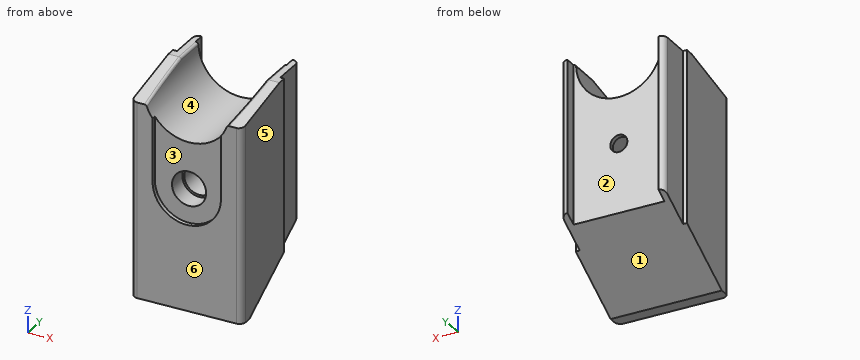
from build123d import *

# Parameters (mm, degrees)
F1_DEPTH  = 26
F2_R      = 10
F2_R_2    = 2
F3_DEPTH  = 26
F4_R      = 3.5
F4_R_2    = 2
F5_DEPTH  = 22.3
F6_R      = 4
F6_R_2    = 3.5
F7_DEPTH  = 5.4
F8_R      = 0.6
F9_W      = 0.9285709113
F9_H      = 8
F10_DEPTH = 61.5
F11_R     = 1.4
F12_W     = 21.2637362675
F12_H     = 42.3296708614
F13_DEPTH = 2.6
F15_DEPTH = 1


with BuildPart() as f1:
    # F0 (on Right) → F1 (new body)
    with BuildSketch(Plane.YZ):
        Polygon((-10, 28.8693108244), (-26, 25.475452911), (-26, -20.1306891756), (-23, -20.1306891756), (0, -6.8516329843), (0, 28.8693108244), align=None)
    extrude(amount=F1_DEPTH)

    # F2 (on face) → F3 (cut)
    with BuildSketch(Plane.XZ.offset(26)):
        with Locations((13, 28.6730788648)):
            Circle(F2_R)
        with Locations((13, 7.8693108244)):
            Circle(F2_R_2)
    extrude(amount=-F3_DEPTH, mode=Mode.SUBTRACT)

    # F4 (on face) → F5 (cut)
    with BuildSketch(Plane.XZ.offset(26)):
        with Locations((13, 7.8693108244)):
            Circle(F4_R)
        with Locations((13, 7.8693108244)):
            Circle(F4_R_2, mode=Mode.SUBTRACT)
    extrude(amount=-F5_DEPTH, mode=Mode.SUBTRACT)

    # F6 (on face) → F7 (cut)
    with BuildSketch(Plane.XZ.offset(26)):
        with Locations((13, 7.8693108244)):
            Circle(F6_R)
        with Locations((13, 7.8693108244)):
            Circle(F6_R_2, mode=Mode.SUBTRACT)
    extrude(amount=-F7_DEPTH, mode=Mode.SUBTRACT)

    # F8
    f8_edges = [f1.edges().sort_by_distance(p)[0] for p in [
        (3.113398, -18.00473, 27.171379),
        (22.999519, -10.462557, 28.771195),
        (22.871208, -18.467044, 27.073314),
        (3.001926, -5, 28.869311),
        (22.998074, -5, 28.869311),
    ]]
    fillet(f8_edges, radius=F8_R)

    # F9 (on face) → F10 (cut)
    with BuildSketch(Plane.XY.offset(28.8693108244)):
        with Locations((25.5357145444, -4)):
            Rectangle(F9_W, F9_H)
        with Locations((0.4642854556, -4)):
            Rectangle(F9_W, F9_H)
    extrude(amount=-F10_DEPTH, mode=Mode.SUBTRACT)

    # F11
    f11_edges = [f1.edges().sort_by_distance(p)[0] for p in [
        (0, -26, 2.672382),
        (26, -26, 2.672382),
        (0.928571, 0, 11.008839),
        (25.071429, 0, 11.008839),
    ]]
    fillet(f11_edges, radius=F11_R)

    # F12 (on face) → F13 (cut)
    with BuildSketch(Plane(origin=(0, 0, 0), x_dir=(-1, 0, 0), z_dir=(0, 1, 0))):
        with Locations((-12.960439045, 10.5494512245)):
            Rectangle(F12_W, F12_H)
    extrude(amount=-F13_DEPTH, mode=Mode.SUBTRACT)

    # F14 (on face) → F15 (cut)
    with BuildSketch(Plane.XZ.offset(26)):
        with BuildLine():
            ThreePointArc((5, 7.9120891169), (13, -0.0879108831), (21, 7.9120891169))
            ThreePointArc((21, 7.9120891169), (13, 15.9120891169), (5, 7.9120891169))
        make_face()
        with BuildLine():
            ThreePointArc((5, 7.9120891169), (13, 15.9120891169), (21, 7.9120891169))
            Line((21, 7.9120891169), (21, 25.7802214473))
            Line((21, 25.7802214473), (5, 25.7802214473))
            Line((5, 25.7802214473), (5, 7.9120891169))
        make_face()
    extrude(amount=-F15_DEPTH, mode=Mode.SUBTRACT)


solid = f1.part
Could you check a few things on this model? Use its own coordinates, in mm. Face numbers are marked on the shaded views. A direction names the side the tool comes from. Give positions to 0.01 mm unless a question says otherwise; leave off trailing zeros. Order: outer loops, then holes, each group sorted by start corner. A loop starts at its lowest first (then second) coordinate and runs counter-clockwise, first axis right, second up. Notation, with made-up numbers: (43.5, -38) - (62.5, -38) arc R20 ccw to (62.5, -24) - close; hole circle Ø11 at (24, -21). An arc over 180 degrees is marked (long way). One line per item, written item: value. Start each with the question number.
1. Imagine slicing it at C-C on y = -4.25. List the corners of the cut face in (x, z) for me, plus the area to 3 significant figures.
2. Imagine slicing it at B-B on z = 24. List the corners of the cut face in (x, y) for me.
3. For P1, Ø4, axis at x = 9, y = -15, coming from the +Z side; P2, Ø2, axis at x = 14.5, z = 6.5, coming from the -Y side; P3, Ø5, axis at x = 13, z = 7.87, coming from the +Y side, each with a flat end and sliding along its axis, tell me the tip position at first contact or that it passes through.
4. If I drill on probe 1 along Y at (x, z) = (15.75, 2); probe 2 along Y at (x, z) = (13, -7); probe 3 along X at (y, z) = (-12, 22), over which ranges is the centre line in solid material (lowest first)?
5. Imagine slicing it at A-A on x = 13. List the corners of the cut face in (y, z) for me, plus the area to 3 significant figures.
6. Thinking about a two-plate mould opening in X: for the marked faces 3, 4, 5 and 6, which applies, +X half, -X half, draft (parallel to the pull), parting line (faces both ways), or undercut?
7. For the marked faces 1 and 2, which set-ups out of +Z, -Z, +X, -X, +Y, -Y let a thin tool reach every point of the face, with its end or its side?
8. Imagine slicing it at D-D on z = 18. List the corners of the cut face in (x, y) for me, plus the area to 3 significant figures.
Values:
1. outline: (0.93, -9.31) - (25.07, -9.31) - (25.07, 28.87) - (23.59, 28.87) arc R0.6 ccw to (22.99, 28.29) arc R10 cw to (3.01, 28.29) arc R0.6 ccw to (2.41, 28.87) - (0.93, 28.87) - close; hole circle Ø7 at (13, 7.87)
1. area: 722 mm²
2. outline: (0, -24.6) arc R1.4 ccw to (1.4, -26) - (4.16, -26) - (4.16, -2.6) - (2.33, -2.6) - (2.33, 0) arc R1.4 ccw to (0.93, -1.4) - (0.93, -8) - (0, -8) - close; (21.84, -26) - (24.6, -26) arc R1.4 ccw to (26, -24.6) - (26, -8) - (25.07, -8) - (25.07, -1.4) arc R1.4 ccw to (23.67, 0) - (23.59, 0) - (23.59, -2.6) - (21.84, -2.6) - close
3. P1: z = 20.67
3. P2: y = -3.7
3. P3: y = -2.6
4. probe 1: -25 to -2.6
4. probe 2: -26 to -2.6
4. probe 3: 0 to 5.55, 20.45 to 26
5. outline: (-26, -20.13) - (-23, -20.13) - (-2.6, -8.35) - (-2.6, 5.87) - (-3.7, 5.87) - (-3.7, 4.37) - (-20.6, 4.37) - (-20.6, 3.87) - (-25, 3.87) - (-25, -0.09) - (-26, -0.09) - close; (-25, 11.87) - (-20.6, 11.87) - (-20.6, 11.37) - (-3.7, 11.37) - (-3.7, 9.87) - (-2.6, 9.87) - (-2.6, 18.67) - (-25, 18.67) - close
5. area: 611 mm²
6. face 3: undercut
6. face 4: undercut
6. face 5: +X half
6. face 6: draft
7. face 1: -Z, +X, -X, +Y
7. face 2: +Z, -Z, +Y
8. outline: (0, -24.6) arc R1.4 ccw to (1.4, -26) - (5, -26) - (5, -25) - (21, -25) - (21, -26) - (24.6, -26) arc R1.4 ccw to (26, -24.6) - (26, -8) - (25.07, -8) - (25.07, -1.4) arc R1.4 ccw to (23.67, 0) - (23.59, 0) - (23.59, -2.6) - (2.33, -2.6) - (2.33, 0) arc R1.4 ccw to (0.93, -1.4) - (0.93, -8) - (0, -8) - close
8. area: 588 mm²
